Source: CAD feature listing. Evaluate the final solid. Frame: model axes, mm. A direction names the side the tool comes from. Give positions to 0.01 mm unless a question says otherwise; leave off trailing zeros. Write each loop counter-clockwise with the first axis right and the second up, starting at its lowest first coordinate (ties: lowest second). Pieces come first, ordered by that corner, then holes. Notation, with made-up numbers: (48, 70.25) -> (87, 70.25) arc R14 ccw to (87, 75.25) -> close; hole circle Ø8 at (42, 18). An arc over 180 degrees is marked (long way). Answer as a JSON object with one key per item and string values. Group by question number.
Item 1: Section query D-D on x = 11.25. Return the cut outline in (y, z), plus the area to 3 significant figures.
Item 2: Section query C-C on z = -1.75. Return the cut outline in (x, y), plus the area to 3 significant figures.
Item 3: Ray query, probe 1 along Y at (x, z) = (15.75, 0.25); probe 2 along X at (y, z) = (-48, -3.75); probe 3 along Y at (x, z) = (17.75, 3.25). Return the intervals inside material, ascending. Write a range as from..to.
Item 4: Pull-direction query (Y, two-part tool) for faces 1 (the face through (1, -47.5, -2)), 2 (the face through (2.5, -49, -2)), 3 (the face through (10, -32.5, 3)); classes: pulls with the +Y half, pulls with the -Y half, needs draft (parallel to the pull), parting line crosses it, or undercut.
Item 5: First-contact query: pin 1 Ø1.1 at (x, y) = (10, -54) entering from +Z; pin 2 Ø0.8 at (y, z) = (-33, 2.5) entering from +X; pin 3 Ø1.2 at (y, z) = (-55.5, 3) entering from -X; pin 4 Ø3 at (y, z) = (-37.5, 4) entering from -X. Flat tips, straight axial feed; report the tip coordinate or a pass-through.
Item 6: Section query A-A on y = -48. Return the cut outline in (x, z), plus the area to 4 significant figures.
Item 7: Section query B-B on x = 2. Return the cut outline in (y, z), plus the area to 3 significant figures.
Item 8: Access query for faces 4 (the face through (1, -42.5, -2)), 5 (the face through (8.2, -35, 0.3)), 6 (the face through (17.5, -41, -2)), 7 (the face through (10, -45, 3)), 8 (the face through (5, -53, 3)). Directions: +Z, -Z, +X, -X, +Y, -Y. A direction counts if a zero-diameter tool reaches every point of the face in a straight line with its end or side. Return the directions, or none.
Autodesk Inventor part; units mm, degrees
ref_plane "YZ Plane" through (0, 0, 0) normal (1, 0, 0) x (0, 1, 0)
ref_plane "XZ Plane" through (0, 0, 0) normal (0, 1, 0) x (-1, 0, 0)
ref_plane "XY Plane" through (0, 0, 0) normal (0, 0, 1) x (1, 0, 0)
sketch "Sketch1" plane through (0, 0, 0) normal (0, 0, 1) x (1, 0, 0)
  line L0 (0, 0) -> (20, 0)
  line L1 (20, 0) -> (20, -2.7984)
  line L2 (0, -2.7984) -> (0, 0)
  line L3 (0, 0) -> (20, 0)
  line L4 (20, 0) -> (20, -50)
  line L5 (20, -50) -> (0, -50)
  line L6 (0, -50) -> (0, 0)
  line L7 (0, 0) -> (5, 0)
  line L8 (0, -5) -> (0, 0)
  circle A0 centre (5, -5) radius 1.651
  line L9 (20, 0) -> (15, 0)
  line L10 (15, -5) -> (20, -5)
  line L11 (20, -5) -> (20, 0)
  circle A1 centre (15, -5) radius 1.651
  dimension "d1" = 20
  dimension "d2" = 50
  dimension "d6" = 5
  dimension "d7" = 5
  dimension "d9" = 3.302
extrude "Extrusion1" add sketch "Sketch1" along normal blind 5
sketch "Sketch2" plane through (0, 0, 5) normal (0, 0, 1) x (1, 0, 0)
  line L0 (20, 0) -> (0, 0)
  line L1 (10, 0) -> (5, 0)
  line L2 (5, 0) -> (5, 5)
  line L3 (5, 5) -> (10, 5)
  line L4 (10, 5) -> (10, 0)
  line L5 (10, 5) -> (2.5, 5)
  line L6 (2.5, 5) -> (2.5, 7.5)
  line L7 (2.5, 7.5) -> (10, 7.5)
  line L8 (10, 7.5) -> (10, 5)
  line L9 (2.5, 7.5) -> (17.5, 7.5)
  line L10 (17.5, 7.5) -> (17.5, 5)
  line L11 (17.5, 5) -> (2.5, 5)
  line L12 (2.5, 5) -> (2.5, 7.5)
  line L13 (10, 5) -> (15, 5)
  line L14 (15, 5) -> (15, 0)
  line L15 (15, 0) -> (10, 0)
  line L16 (10, 0) -> (10, 5)
  dimension "d12" = 5
  dimension "d13" = 5
  dimension "d14" = 7.5
  dimension "d15" = 2.5
  dimension "d16" = 15
  dimension "d17" = 2.5
  dimension "d18" = 5
  dimension "d19" = 5
extrude "Extrusion2" add sketch "Sketch2" against normal blind 5
sketch "Sketch3" plane through (0, 0, 0) normal (0, 0, -1) x (-1, 0, 0)
  line L0 (-5, 0) -> (-5, 5)
  line L1 (-5, 0) -> (-15, 0)
  line L2 (-15, 0) -> (-15, 5)
  line L3 (-15, 5) -> (-5, 5)
  line L4 (-5, 5) -> (-5, 0)
  point P0 (0, 0)
extrude "Extrusion3" cut sketch "Sketch3" against normal blind 1
sketch "Sketch4" plane through (0, 0, 0) normal (0, 0, -1) x (-1, 0, 0)
  line L0 (-5, 0) -> (0, 0)
  line L1 (-20, -50) -> (0, -50)
  line L2 (0, 0) -> (-20, 0)
  line L3 (-20, 0) -> (-20, -50)
  line L4 (-20, -50) -> (0, -50)
  line L5 (0, -50) -> (0, 0)
  line L6 (0, -50) -> (-5, -50)
  line L7 (-5, -50) -> (-5, -30)
  line L8 (-5, -30) -> (0, -30)
  line L9 (0, -30) -> (0, -50)
  line L10 (0, -50) -> (0, 0)
  line L11 (0, -50) -> (-5, -50)
  line L12 (-5, -50) -> (-5, -30)
  line L13 (-5, -30) -> (0, -30)
  line L14 (0, -30) -> (0, -50)
  line L15 (0, -50) -> (-20, -50)
  line L16 (-20, -50) -> (-20, -45)
  line L17 (-20, -45) -> (0, -45)
  line L18 (0, -45) -> (0, -50)
  dimension "d28" = 5
  dimension "d29" = 20
  dimension "d30" = 5
  dimension "d31" = 20
  dimension "d32" = 20
  dimension "d33" = 5
extrude "Extrusion4" add sketch "Sketch4" along normal blind 15 contours L17 L7 L1 L3 | L5 L1 L7 L17
sketch "Sketch5" plane through (0, 0, 5) normal (0, 0, 1) x (1, 0, 0)
  line L0 (20, -50) -> (20, 0)
  line L1 (20, 0) -> (0, 0)
  line L2 (0, 0) -> (0, -50)
  line L3 (0, -50) -> (20, -50)
  line L4 (20, -50) -> (20, 0)
  line L5 (10, -50) -> (15, -50)
  line L6 (15, -50) -> (15, -55)
  line L7 (15, -55) -> (10, -55)
  line L8 (10, -55) -> (10, -50)
  line L9 (15, -55) -> (5, -55)
  line L10 (5, -55) -> (5, -50)
  line L11 (5, -50) -> (15, -50)
  line L12 (15, -50) -> (15, -55)
  line L13 (10, -55) -> (17.5, -55)
  line L14 (17.5, -55) -> (17.5, -57.5)
  line L15 (17.5, -57.5) -> (10, -57.5)
  line L16 (10, -57.5) -> (10, -55)
  line L17 (17.5, -57.5) -> (2.5, -57.5)
  line L18 (2.5, -57.5) -> (2.5, -55)
  line L19 (2.5, -55) -> (17.5, -55)
  line L20 (17.5, -55) -> (17.5, -57.5)
  dimension "d36" = 5
  dimension "d37" = 5
  dimension "d38" = 10
  dimension "d39" = 5
  dimension "d40" = 7.5
  dimension "d41" = 2.5
  dimension "d42" = 15
  dimension "d43" = 2.5
extrude "Extrusion5" add sketch "Sketch5" against normal blind 5 contours L6 L7 L8 L3 | L8 L9 L10 L3 | L13 L14 L15 L16 L7 | L16 L17 L18 L19 L9
sketch "Sketch6" plane through (0, 0, 0) normal (0, 0, -1) x (-1, 0, 0)
  line L0 (-5, -55) -> (-5, -50)
  line L1 (-15, -50) -> (-5, -50)
  line L2 (-5, -55) -> (-15, -55)
  line L3 (-15, -55) -> (-15, -50)
  line L4 (-15, -50) -> (-5, -50)
  line L5 (-5, -50) -> (-5, -55)
  point P0 (0, 0)
extrude "Extrusion6" cut sketch "Sketch6" against normal blind 1
sketch "Sketch8" plane through (0, -45, 0) normal (0, 1, 0) x (1, 0, 0)
  line L0 (0, 15) -> (20, 15)
  line L1 (0, 15) -> (20, 15)
  line L2 (20, 15) -> (20, 0)
  line L3 (20, 0) -> (0, 0)
  line L4 (0, 0) -> (0, 15)
  line L5 (0, 0) -> (0, 15)
  line L6 (0, 7.5) -> (20, 7.5)
  line L7 (20, 0) -> (20, 15)
  line L8 (20, 0) -> (0, 15)
  line L9 (20, 15) -> (0, 0)
  line L10 (10, 7.5) -> (10, 15)
  line L11 (10, 7.5) -> (10, 0)
  line L12 (10, 7.5) -> (0, 0)
  line L13 (10, 7.5) -> (20, 0)
  line L14 (10, 7.5) -> (0, 15)
  line L15 (10, 7.5) -> (20, 15)
  circle A0 centre (5, 3.75) radius 1.651
  circle A1 centre (15, 3.75) radius 1.651
  circle A2 centre (15, 11.25) radius 1.651
  circle A3 centre (5, 11.25) radius 1.651
  dimension "d48" = 3.302
  dimension "d49" = 3.302
  dimension "d50" = 3.302
  dimension "d51" = 3.302
extrude "Extrusion7" cut sketch "Sketch8" against normal blind 5 contours A3 L8 | L8 A3 | A2 L9 | L9 A2 | A1 L8 | L8 A1 | A0 L9 | L9 A0
sketch "Sketch9" plane through (0, 0, 0) normal (0, 0, -1) x (-1, 0, 0)
  line L0 (6.3074, -39.8098) -> (-37.7059, -39.8098)
  line L1 (-37.7059, -39.8098) -> (-37.7059, -53.6211)
  line L2 (-37.7059, -53.6211) -> (6.3074, -53.6211)
  line L3 (6.3074, -53.6211) -> (6.3074, -39.8098)
  point P0 (0, 0)
extrude "Extrusion8" cut sketch "Sketch9" along normal blind 100
sketch "Sketch10" plane through (0, 0, 0) normal (0, 0, -1) x (-1, 0, 0)
  line L0 (0, 0) -> (0, -50)
  line L1 (-20, -50) -> (-20, 0)
  line L2 (0, -50) -> (-20, -50)
  line L3 (-20, -50) -> (-20, -40)
  line L4 (-20, -40) -> (0, -40)
  line L5 (0, -40) -> (0, -50)
  line L6 (-20, -40) -> (0, -40)
  line L7 (0, -40) -> (0, 19.6469)
  line L8 (0, 19.6469) -> (-20, 19.6469)
  line L9 (-20, 19.6469) -> (-20, -40)
  dimension "d56" = 10
extrude "Extrusion9" cut sketch "Sketch10" against normal blind 100 contours L0 L4 L1 L9 L8 L7
sketch "Sketch11" plane through (0, 0, 5) normal (0, 0, 1) x (1, 0, 0)
  line L0 (0, -40) -> (20, -40)
  line L1 (10, -40) -> (15, -40)
  line L2 (15, -40) -> (15, -35)
  line L3 (15, -35) -> (10, -35)
  line L4 (10, -35) -> (10, -40)
  line L5 (10, -35) -> (17.5, -35)
  line L6 (17.5, -35) -> (17.5, -32.5)
  line L7 (17.5, -32.5) -> (10, -32.5)
  line L8 (10, -32.5) -> (10, -35)
  line L9 (17.5, -32.5) -> (2.5, -32.5)
  line L10 (2.5, -32.5) -> (2.5, -35)
  line L11 (2.5, -35) -> (17.5, -35)
  line L12 (17.5, -35) -> (17.5, -32.5)
  line L13 (10, -35) -> (5, -35)
  line L14 (5, -35) -> (5, -40)
  line L15 (5, -40) -> (10, -40)
  line L16 (10, -40) -> (10, -35)
  point P0 (0, 0)
  dimension "d59" = 5
  dimension "d60" = 5
  dimension "d61" = 7.5
  dimension "d62" = 2.5
  dimension "d63" = 15
  dimension "d64" = 2.5
  dimension "d65" = 5
  dimension "d66" = 5
extrude "Extrusion10" add sketch "Sketch11" against normal blind 5
sketch "Sketch12" plane through (0, 0, 0) normal (0, 0, -1) x (-1, 0, 0)
  line L0 (-15, -35) -> (-15, -40)
  line L1 (-5, -40) -> (0, -40)
  line L2 (-15, -35) -> (-5, -35)
  line L3 (-5, -35) -> (-5, -40)
  line L4 (-5, -40) -> (-15, -40)
  line L5 (-15, -40) -> (-15, -35)
  point P0 (0, 0)
extrude "Extrusion11" cut sketch "Sketch12" against normal blind 1
sketch "Sketch13" plane through (20, -50, 5) normal (1, 0, 0) x (0, 0, -1)
  line L0 (5, 10) -> (0, 10)
  line L1 (0, 0) -> (5, 0)
  line L2 (5, 10) -> (0, 10)
  line L3 (0, 10) -> (0, 0)
  line L4 (0, 0) -> (5, 0)
  line L5 (5, 0) -> (5, 10)
  line L6 (0, 0) -> (0, 10)
  line L7 (0, 5) -> (2, 5)
  line L8 (2, 5) -> (2, 2.5)
  line L9 (2, 2.5) -> (0, 2.5)
  line L10 (0, 2.5) -> (0, 5)
  line L11 (2, 2.5) -> (0, 2.5)
  line L12 (0, 2.5) -> (0, 7.5)
  line L13 (0, 7.5) -> (2, 7.5)
  line L14 (2, 7.5) -> (2, 2.5)
  point P0 (5, 50)
  dimension "d71" = 2
  dimension "d72" = 2.5
  dimension "d73" = 5
extrude "Extrusion12" cut sketch "Sketch13" against normal blind 20 contours L13 L14 L7 L3 | L7 L8 L9 L3
sketch "Sketch14" plane through (0, 0, 0) normal (0, 0, -1) x (-1, 0, 0)
  line L0 (-20, -40) -> (-15, -40)
  line L1 (-20, -40) -> (-17.5, -40)
  line L2 (-17.5, -40) -> (-17.5, -42.5)
  line L3 (-17.5, -42.5) -> (-20, -42.5)
  line L4 (-20, -42.5) -> (-20, -40)
  line L5 (-15, -50) -> (-20, -50)
  line L6 (-20, -50) -> (-17.5, -50)
  line L7 (-17.5, -50) -> (-17.5, -47.5)
  line L8 (-17.5, -47.5) -> (-20, -47.5)
  line L9 (-20, -47.5) -> (-20, -50)
  line L10 (0, -50) -> (0, -40)
  line L11 (0, -40) -> (-2.5, -40)
  line L12 (-2.5, -40) -> (-2.5, -42.5)
  line L13 (-2.5, -42.5) -> (0, -42.5)
  line L14 (0, -42.5) -> (0, -40)
  line L15 (0, -50) -> (-2.5, -50)
  line L16 (-2.5, -50) -> (-2.5, -47.5)
  line L17 (-2.5, -47.5) -> (0, -47.5)
  line L18 (0, -47.5) -> (0, -50)
  point P0 (0, 0)
  dimension "d76" = 2.5
  dimension "d77" = 2.5
  dimension "d78" = 2.5
  dimension "d79" = 2.5
  dimension "d80" = 2.5
  dimension "d81" = 2.5
  dimension "d82" = 2.5
  dimension "d83" = 2.5
extrude "Extrusion13" add sketch "Sketch14" along normal blind 5
sketch "Sketch15" plane through (2.5, -57.5, 5) normal (0, -1, 0) x (1, 0, 0)
  line L0 (17.5, 0) -> (-2.5, 0)
  line L1 (7.5, 0) -> (7, 0)
  line L2 (7, 0) -> (7, -0.5)
  line L3 (7, -0.5) -> (7.5, -0.5)
  line L4 (7.5, -0.5) -> (7.5, 0)
  line L5 (7, 0) -> (8, 0)
  line L6 (8, 0) -> (8, -0.5)
  line L7 (8, -0.5) -> (7, -0.5)
  line L8 (7, -0.5) -> (7, 0)
  point P0 (-2.5, -5)
  dimension "d86" = 0.5
  dimension "d87" = 0.5
  dimension "d88" = 1
  dimension "d89" = 0.5
extrude "Extrusion14" cut sketch "Sketch15" against normal blind 500
properties part number "CableGuide"
Worked answers:
{
 "1": {"outline": "(-57.5, 0) -> (-55, 0) -> (-55, 1) -> (-50, 1) -> (-50, 0) -> (-40, 0) -> (-40, 1) -> (-35, 1) -> (-35, 0) -> (-32.5, 0) -> (-32.5, 5) -> (-42.5, 5) -> (-42.5, 3) -> (-47.5, 3) -> (-47.5, 5) -> (-57.5, 5) -> close", "area": "105 mm^2"},
 "2": {"outline": "(0, -50) -> (2.5, -50) -> (2.5, -47.5) -> (0, -47.5) -> close; (0, -42.5) -> (2.5, -42.5) -> (2.5, -40) -> (0, -40) -> close; (17.5, -50) -> (20, -50) -> (20, -47.5) -> (17.5, -47.5) -> close; (17.5, -42.5) -> (20, -42.5) -> (20, -40) -> (17.5, -40) -> close", "area": "25.0 mm^2"},
 "3": {"probe 1": "-57.5..-55, -50..-40, -35..-32.5", "probe 2": "0..2.5, 17.5..20", "probe 3": "-50..-47.5, -42.5..-40"},
 "4": {"face 1": "undercut", "face 2": "needs draft", "face 3": "pulls with the +Y half"},
 "5": {"pin 1": "z = 5", "pin 2": "x = 17.5", "pin 3": "x = 2.5", "pin 4": "x = 5"},
 "6": {"outline": "(0, -5) -> (2.5, -5) -> (2.5, 0) -> (17.5, 0) -> (17.5, -5) -> (20, -5) -> (20, 5) -> (10.5, 5) -> (10.5, 4.5) -> (9.5, 4.5) -> (9.5, 5) -> (0, 5) -> close", "area": "124.5 mm^2"},
 "7": {"outline": "(-50, -5) -> (-47.5, -5) -> (-47.5, 0) -> (-42.5, 0) -> (-42.5, -5) -> (-40, -5) -> (-40, 5) -> (-42.5, 5) -> (-42.5, 3) -> (-47.5, 3) -> (-47.5, 5) -> (-50, 5) -> close", "area": "65.0 mm^2"},
 "8": {"face 4": "-Z, +X, -X", "face 5": "-Z", "face 6": "-Z, +Y, -Y", "face 7": "+Z, +X, -X", "face 8": "+Z, -Z, -X"}
}
